from build123d import *

# Parameters (mm, degrees)
ESQUISSE1_W             = 22
ESQUISSE1_H             = 22
BASE_EXTRUSION_DEPTH    = 298
ESQUISSE2_R             = 3.375
ENL_V_MAT_EXTRU_1_DEPTH = 25
ENL_V_START             = -25
ESQUISSE3_R             = 3.375
ENL_V_MAT_EXTRU_2_DEPTH = 25


with BuildPart() as part:
    # Esquisse1 → Base-Extrusion (new body)
    with BuildSketch(Plane.XY):
        with Locations((11, 11)):
            Rectangle(ESQUISSE1_W, ESQUISSE1_H)
    extrude(amount=BASE_EXTRUSION_DEPTH)

    # Esquisse2 → Enlèv. mat.-Extru.1 (cut)
    with BuildSketch(Plane.XY.offset(298)):
        with Locations((11, 11)):
            Circle(ESQUISSE2_R)
    extrude(amount=-ENL_V_MAT_EXTRU_1_DEPTH, mode=Mode.SUBTRACT)

    # Esquisse3 → Enlèv. mat.-Extru.2 (cut)
    with BuildSketch(Plane(origin=(0, 0, 0), x_dir=(-1, 0, 0), z_dir=(0, 0, -1)).offset(ENL_V_START)):
        with Locations(Location((-11, 11, 0), (0, 0, 180))):
            Circle(ESQUISSE3_R)
    extrude(amount=ENL_V_MAT_EXTRU_2_DEPTH, mode=Mode.SUBTRACT)


solid = part.part
The model under review builds one solid part; all positions refer to its coordinate system, in mm. A direction names the side the tool comes from. Coordinates: 2 decimals unless noted, no trailing zeros. Loops run counter-clockwise (first coordinate to the right, second up) from the corner with the lowest first, then second, coordinate; pieces in that order, holes last. Notation, with made-up numbers: M -36.75,32 L 11.25,32 A26 ccw 11.25,70 Z; hole C 65,-29 d11. An arc over 180 degrees is marked long. Put each result on its own line as item: value. Start each with the question number.
Q1. Add section B-B (z = 18). Write out the cut boundary in (x, y) (3 decimals), and give its area (3 significant figures).
Q2. Wall thickness on line 1 (Y direction, x = 11, z = 282) (3 decimals): over which ranges is the line inside the solid? List them lowest first.
Q3. The part is to be moulded in two halves that separate along X. For faces 1 (the cylindrical face through (12.81, 13.85, 285.68)), 2 (the flat face through (22, 11, 147)), 3 (the cylindrical face through (12.557, 13.994, 12.675)), 4 (the flat face through (11, 0, 147)), say which applies: +X half, -X half, draft (parallel to the pull), parting line (faces both ways), or undercut.
Q4. Clearance check with flat-ended pins moving along their axes: pin 1 (2 mm diameter, centred on x = 11, y = 10, fed in from +Z); pin 2 (6 mm diameter, centred on x = 11, y = 11, fed in from -Z). State where each tip first meets the part, or that it passes through.
Q5. Add section A-A (y = 11). Write out the cut boundary in (x, z) (3 decimals), and give its area (3 significant figures).
Q6. For faces 5 (the flat face through (11, 11, 25)), 6 (the flat face through (8, 14, 298)), 7 (the flat face through (11, 11, 273)), list the 3-axis set-ups (+Z, -Z, +X, -X, +Y, -Y) from which the entire face can be reached by the end or side of a thin tool; tool diameter is ignored.
Answers:
1. outline: M 0,0 L 22,0 L 22,22 L 0,22 Z; hole C 11,11 d6.75
1. area: 448 mm^2
2. line 1: y = 0 to 7.625, 14.375 to 22
3. face 1: undercut
3. face 2: +X half
3. face 3: undercut
3. face 4: draft
4. pin 1: stops at z = 273
4. pin 2: stops at z = 25
5. outline: M 0,0 L 7.625,0 L 7.625,25 L 14.375,25 L 14.375,0 L 22,0 L 22,298 L 14.375,298 L 14.375,273 L 7.625,273 L 7.625,298 L 0,298 Z
5. area: 6,220 mm^2
6. face 5: -Z
6. face 6: +Z, +X, -X, +Y, -Y
6. face 7: +Z
